from build123d import *

# Parameters (mm, degrees)
BOSS_EXTRUDE1_DEPTH = 82.55
CUT_EXTRUDE1_DEPTH  = 50.8
FILLET1_R           = 6.35
SKETCH3_W           = 18.816678221
SKETCH3_H           = 21.85775753
CUT_EXTRUDE2_DEPTH  = 101.6
CUT_EXTRUDE3_DEPTH  = 50.8
SKETCH5_R           = 1.5875
CUT_EXTRUDE4_DEPTH  = 25.4
SKETCH6_R           = 1.5875
CUT_EXTRUDE5_DEPTH  = 10.16


with BuildPart() as part:
    # Sketch1 → Boss-Extrude1 (new body)
    with BuildSketch(Plane.XY):
        Polygon((-20.934516129, 0), (55.265483871, 0), (55.265483871, 35.8775), (50.820483871, 35.8775), (46.375483871, 6.35), (-12.044516129, 6.35), (-16.489516129, 35.8775), (-20.934516129, 35.8775), align=None)
    extrude(amount=BOSS_EXTRUDE1_DEPTH)

    # Sketch2 → Cut-Extrude1 (cut)
    with BuildSketch(Plane(origin=(0, 35.8775, 0), x_dir=(1, 0, 0), z_dir=(0, 1, 0))):
        Polygon((-1.884516129, -53.975), (-1.884516129, -28.575), (-1.884516129, -16.51), (-20.934516129, -16.51), (-20.934516129, -67.31), (-1.884516129, -67.31), align=None)
    extrude(amount=-CUT_EXTRUDE1_DEPTH, mode=Mode.SUBTRACT)

    # Fillet1
    fillet1_edges = [part.edges().sort_by_distance(p)[0] for p in [
        (-1.884516129, 3.175, 16.51),
        (-1.884516129, 3.175, 67.31),
    ]]
    fillet(fillet1_edges, radius=FILLET1_R)

    # Sketch3 → Cut-Extrude2 (cut)
    with BuildSketch(Plane.XY.offset(82.55)):
        with Locations((52.042862191, 29.978878765)):
            Rectangle(SKETCH3_W, SKETCH3_H)
    extrude(amount=-CUT_EXTRUDE2_DEPTH, mode=Mode.SUBTRACT)

    # Sketch4 → Cut-Extrude3 (cut)
    with BuildSketch(Plane.XZ):
        Polygon((13.990483871, 63.5), (39.390483871, 63.5), (26.690483871, 44.45), align=None)
        Polygon((10.815483871, 61.595), (24.362150538, 41.275), (10.815483871, 20.955), align=None)
        Polygon((42.565483871, 61.595), (42.565483871, 20.955), (29.442150538, 41.275), align=None)
        Polygon((13.990483871, 19.05), (26.690483871, 38.1), (39.390483871, 19.05), align=None)
    extrude(amount=-CUT_EXTRUDE3_DEPTH, mode=Mode.SUBTRACT)

    # Sketch5 → Cut-Extrude4 (cut)
    with BuildSketch(Plane.ZY.offset(20.934516129)):
        with Locations(Location((7.9375, 16.51, 0), (0, 0, 270))):
            Circle(SKETCH5_R)
        with Locations(Location((74.6125, 16.51, 0), (0, 0, 270))):
            Circle(SKETCH5_R)
    extrude(amount=-CUT_EXTRUDE4_DEPTH, mode=Mode.SUBTRACT)

    # Sketch6 → Cut-Extrude5 (cut)
    with BuildSketch(Plane(origin=(55.265483871, 0, 0), x_dir=(0, 0, -1), z_dir=(1, 0, 0))):
        with Locations((-9.525, 9.525)):
            Circle(SKETCH6_R)
        with Locations((-73.025, 9.525)):
            Circle(SKETCH6_R)
    extrude(amount=-CUT_EXTRUDE5_DEPTH, mode=Mode.SUBTRACT)


solid = part.part
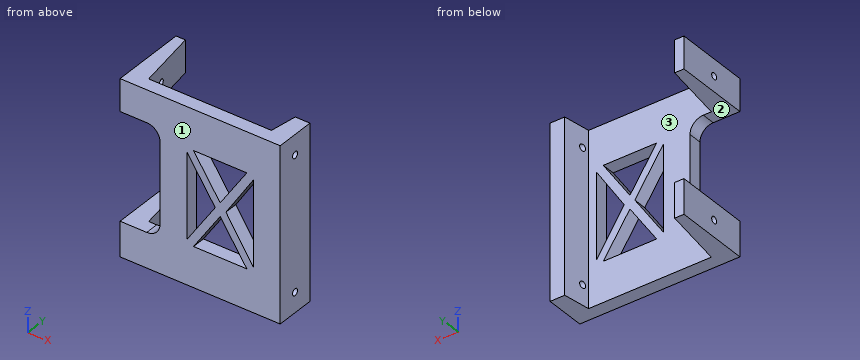
Here's how the part is built. I have some questions about the finished solid (model axes, mm). Face numbers are marked on the shaded views. A direction names the side the tool comes from. Coordinates: 2 decimals unless noted, no trailing zeros. Loops run counter-clockwise (first coordinate to the right, second up) from the corner with the lowest first, then second, coordinate; pieces in that order, holes last. Notation, with made-up numbers: (80.5, -10) -> (121.5, -10) arc R36 cw to (121.5, 26) -> close; hole circle Ø6 at (43.5, 46.5). An arc over 180 degrees is marked (long way). Use one line per item in the form item = value. Start each with the question number.
(1) If we section it at C-C (y = 16.51): Please give me the cut outline in (x, z) (3 decimals).
(2) If we section it at B-B (z = 29): Please give me the cut outline in (x, y), then the cut area to 3 significant figures.
(3) If we section it at D-D (x = 20): Please give me the cut outline in (y, z).
(4) On a 3-axis mill with a long thin cutter (end or side, diameter ignored), from which of +Z, -Z, +X, -X, +Y, -Y can I reach the whole of each face in a straight line? I mean the marked faces 1, 2 and 3. Say none if no direction works.
(5) Will these pins go through, and if not, where does the flat tip stop? pin 1 (7 mm diameter, centred on y = 3, z = 49.5, fed in from -X); pin 2 (3.5 mm diameter, centred on x = 51.5, z = 47, fed in from +Y); pin 3 (2.5 mm diameter, centred on y = 16.51, z = 7.94, fed in from -X).
(6) Please list where these lines run through material, in increasing order: line 1 along Z through (x, y) = (-18.5, 16.51) (3 decimals); line 2 along Z through (x, y) = (38, 2.5); line 3 along Z through (x, y) = (-15, 18.5).
(7) If we section it at A-A (y = 5): Please give me the cut outline in (x, z) (3 decimals).
Verdict:
q1.outline = (-20.935, 0) -> (-13.574, 0) -> (-13.574, 6.35) -> (-20.935, 6.35) -> close; (-20.935, 9.525) -> (-13.574, 9.525) -> (-13.574, 16.51) -> (-20.935, 16.51) -> close; (-20.935, 67.31) -> (-13.574, 67.31) -> (-13.574, 73.025) -> (-20.935, 73.025) -> close; (-20.935, 76.2) -> (-13.574, 76.2) -> (-13.574, 82.55) -> (-20.935, 82.55) -> close; (47.905, 0) -> (55.265, 0) -> (55.265, 82.55) -> (47.905, 82.55) -> close
q2.outline = (-1.88, 0) -> (10.82, 0) -> (10.82, 6.35) -> (-1.88, 6.35) -> close; (16.18, 0) -> (20.62, 0) -> (20.62, 6.35) -> (16.18, 6.35) -> close; (32.76, 0) -> (37.37, 0) -> (37.37, 6.35) -> (32.76, 6.35) -> close; (42.57, 0) -> (55.27, 0) -> (55.27, 19.05) -> (48.29, 19.05) -> (46.38, 6.35) -> (42.57, 6.35) -> close
q2.area = 320 mm²
q3.outline = (0, 0) -> (6.35, 0) -> (6.35, 19.05) -> (0, 19.05) -> close; (0, 28.06) -> (6.35, 28.06) -> (6.35, 34.73) -> (0, 34.73) -> close; (0, 47.82) -> (6.35, 47.82) -> (6.35, 54.49) -> (0, 54.49) -> close; (0, 63.5) -> (6.35, 63.5) -> (6.35, 82.55) -> (0, 82.55) -> close
q4.face_1 = +Z, -Z, +X, -X, -Y
q4.face_2 = -X, +Y, -Y
q4.face_3 = +Z, -Z, +Y
q5.pin_1 = -1.88
q5.pin_2 = 19.05
q5.pin_3 = 47.72
q6.line_1 = 0 to 6.35, 9.525 to 16.51, 67.31 to 73.025, 76.2 to 82.55
q6.line_2 = 0 to 19.05, 21.14 to 28.02, 54.53 to 61.41, 63.5 to 82.55
q6.line_3 = 0 to 16.51, 67.31 to 82.55
q7.outline = (-20.935, 0) -> (55.265, 0) -> (55.265, 82.55) -> (-20.935, 82.55) -> (-20.935, 67.31) -> (-8.235, 67.31) arc R6.35 cw to (-1.885, 60.96) -> (-1.885, 22.86) arc R6.35 cw to (-8.235, 16.51) -> (-20.935, 16.51) -> close; hole (10.815, 20.955) -> (24.362, 41.275) -> (10.815, 61.595) -> close; hole (13.99, 19.05) -> (39.39, 19.05) -> (26.69, 38.1) -> close; hole (13.99, 63.5) -> (26.69, 44.45) -> (39.39, 63.5) -> close; hole (29.442, 41.275) -> (42.565, 20.955) -> (42.565, 61.595) -> close
